Could you check a few things on this drawing? It's one solid part, dimensions in mm from its lowest x, y, z. Coordinates: 2 decimals unless noted, no trailing zeros. Write each loop counter-clockwise with the first axis right and the second up, starting at its lowest first coordinate (ties: lowest second). Pieces come first, ordered by that corner, then holes.
Item 1: I'm going to push flat-ended pins straight in: P1, Ø1.6, axis at x = 3.65, z = 9.6, coming from the +Y side; P2, Ø1, axis at x = 5.5, z = 19, coming from the -Y side; P3, Ø2.5, axis at x = 3.5, z = 2.5, coming from the +Y side. Where does each tip first touch, or does it pass through?
Item 2: I want a section at C-C (x = 5.5). Please give me the cut outline in (y, z) (1 decimal), and give its area (3 significant figures).
Item 3: I want a section at A-A (z = 3.65). Please give me the cut outline in (x, y).
Item 4: I want a section at B-B (y = 3.7). Please give me the cut outline in (x, z), and give its area (3 significant figures).
Item 5: If we mould it in two halves opening along X, with no side actions, what happens to the marked faces 1, 2 and 3? For each: pulls with the +X half, pulls with the -X half, needs draft (parallel to the pull), parting line crosses it, or undercut.
Item 6: Please list where these lines run through material, in increasing order: line 1 (X direction, y = 2.65, z = 19.6); line 2 (Y direction, x = 2.75, z = 15.5); line 3 (Y direction, x = 5.5, z = 2.25).
Item 7: I want a section at D-D (z = 12.1). Please give me the cut outline in (x, y), and give its area (3 significant figures).
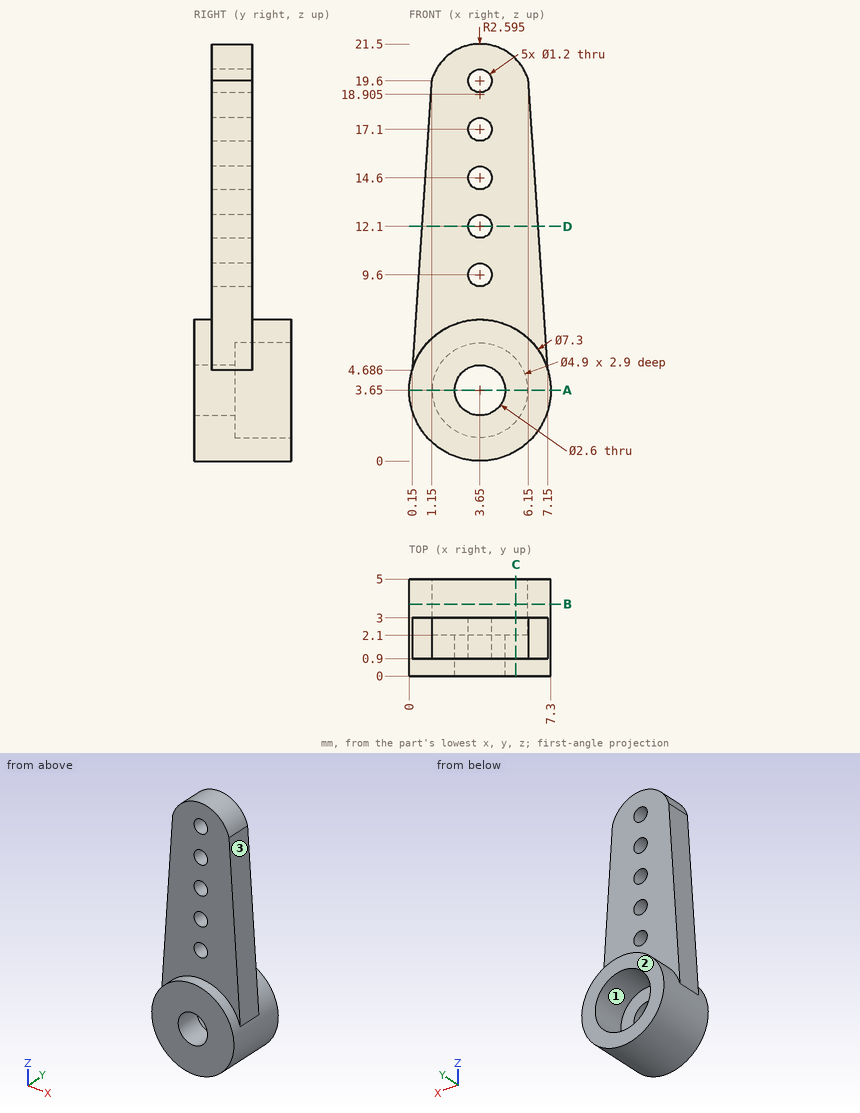
Answer:
1. P1: stops at y = 3
1. P2: stops at y = 0.9
1. P3: stops at y = 2.1
2. outline: (0, 0.5) - (5, 0.5) - (5, 2) - (2.1, 2) - (2.1, 5.3) - (5, 5.3) - (5, 6.8) - (3, 6.8) - (3, 20.7) - (0.9, 20.7) - (0.9, 6.8) - (0, 6.8) - close
2. area: 51.4 mm2
3. outline: (0, 0) - (2.35, 0) - (2.35, 2.1) - (1.2, 2.1) - (1.2, 5) - (0, 5) - close; (4.95, 0) - (7.3, 0) - (7.3, 5) - (6.1, 5) - (6.1, 2.1) - (4.95, 2.1) - close
4. outline: circle Ø7.3 at (3.65, 3.65); hole circle Ø4.9 at (3.65, 3.65)
4. area: 23.0 mm2
5. face 1: undercut
5. face 2: needs draft
5. face 3: pulls with the +X half
6. line 1: x = 1.15 to 3.05, 4.25 to 6.15
6. line 2: y = 0.9 to 3
6. line 3: y = 0 to 2.1
7. outline: (0.65, 0.9) - (3.05, 0.9) - (3.05, 3) - (0.65, 3) - close; (4.25, 0.9) - (6.65, 0.9) - (6.65, 3) - (4.25, 3) - close
7. area: 10.1 mm2
